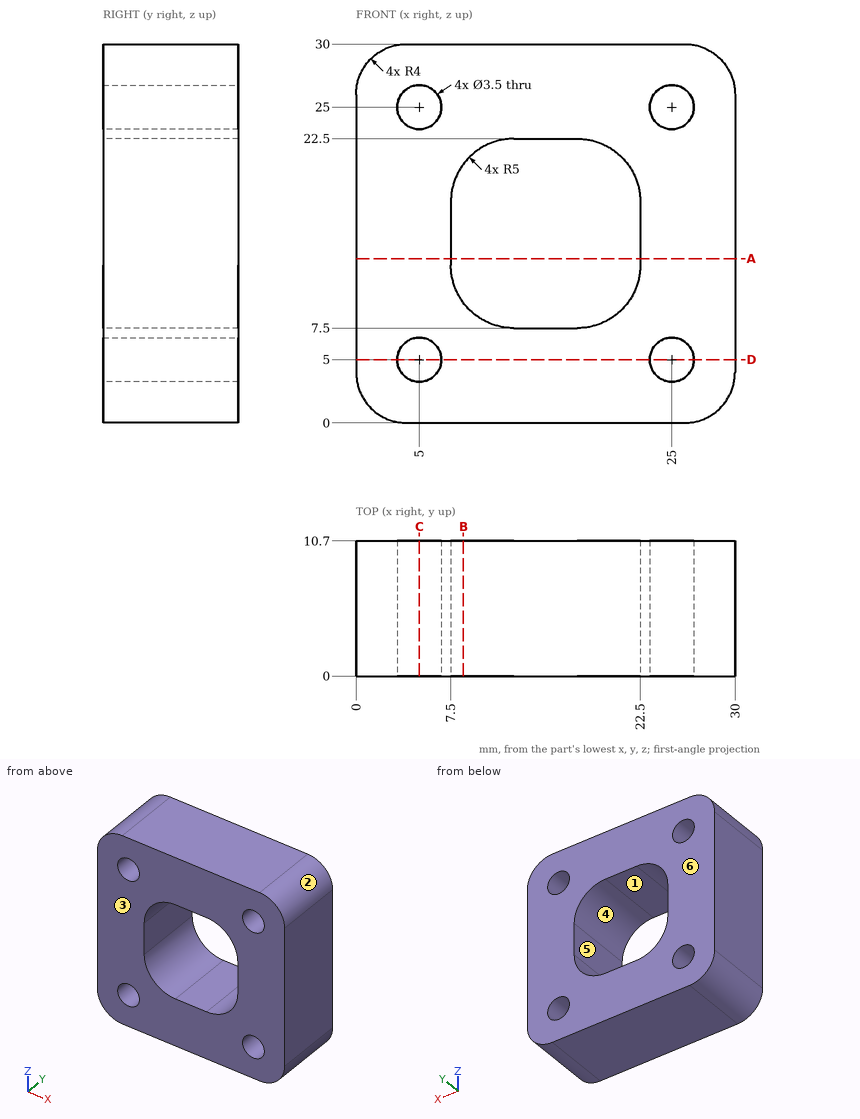
Geometry check sheet. Reference: drawing and pictorial views, mm from the part's lowest x, y, z. A direction names the side the tool comes from. Give positions to 0.01 mm unless a question says otherwise; leave off trailing zeros. Order: outer loops, then holes, each group sorted by start corner. A loop starts at its lowest first (then second) coordinate and runs counter-clockwise, first axis right, second up. Notation, with made-up numbers: M 41.25,3 L 56.25,3 A23 ccw 56.25,21 Z; hole C 86,-9 d9. An arc over 180 degrees is marked long. Answer in a Markdown table with one row per item. Add a question column.
Q1. Sectioned sample at C-C, the plane x = 5. Record the boundary of the cut face in (y, z).
Q2. Sectioned sample at A-A, the plane z = 13. Record the boundary of the cut face in (x, y).
Q3. Thickness scan on L1, parallel to Z at x = 25, y = 5; L2, parallel to Z at x = 26, y = 8.75. Record the ranges inside material, lowest first.
Q4. Release check for a two-part mould opening along Z. For the marked faces 1, 2, 3 and 4 record: released by +Z, released by -Z, zero draft, split by the parting line, or undercut.
Q5. Sectioned sample at B-B, the plane x = 8.5. Record the boundary of the cut face in (y, z), and give its area (3 significant figures).
Q6. Access from +Z, -Z, +X, -X, +Y, -Y to the whole of each face (thin tool, end or side, straight path). Record for the marked faces 5 and 6.
Q7. Gauge pin test, flat ends, axial feed: pin 1 Ø2 at (x, z) = (5, 25) entering from +Y; pin 2 Ø5.5 at (y, z) = (5, 14) entering from -X. Record the tip position at first contact, or that the pin passes through.
Q8. Sectioned sample at D-D, the plane z = 5. Record the boundary of the cut face in (x, y).
Verdict:
| question | item | result |
|---|---|---|
| 1 | outline | M 0,0 L 10.7,0 L 10.7,3.25 L 0,3.25 Z; M 0,6.75 L 10.7,6.75 L 10.7,23.25 L 0,23.25 Z; M 0,26.75 L 10.7,26.75 L 10.7,30 L 0,30 Z |
| 2 | outline | M 0,0 L 7.5,0 L 7.5,10.7 L 0,10.7 Z; M 22.5,0 L 30,0 L 30,10.7 L 22.5,10.7 Z |
| 3 | L1 | 0 to 3.25, 6.75 to 23.25, 26.75 to 30 |
| 3 | L2 | 0 to 3.56, 6.44 to 23.56, 26.44 to 30 |
| 4 | face 1 | undercut |
| 4 | face 2 | released by +Z |
| 4 | face 3 | zero draft |
| 4 | face 4 | undercut |
| 5 | outline | M 0,0 L 10.7,0 L 10.7,9.5 L 0,9.5 Z; M 0,20.5 L 10.7,20.5 L 10.7,30 L 0,30 Z |
| 5 | area | 203 mm² |
| 6 | face 5 | +Y, -Y |
| 6 | face 6 | +Z, -Z, +X, -X, +Y |
| 7 | pin 1 | through |
| 7 | pin 2 | x = 0 |
| 8 | outline | M 0,0 L 3.25,0 L 3.25,10.7 L 0,10.7 Z; M 6.75,0 L 23.25,0 L 23.25,10.7 L 6.75,10.7 Z; M 26.75,0 L 30,0 L 30,10.7 L 26.75,10.7 Z |
